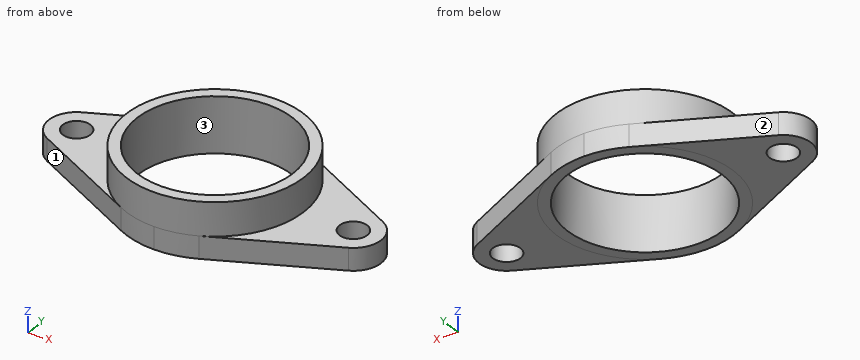
from build123d import *

# Parameters (mm, degrees)
SKETCH_R     = 5
PAD_DEPTH    = 8
SKETCH001_R  = 32
PAD001_DEPTH = 20
SKETCH002_R  = 28
POCKET_DEPTH = 20.0010001


with BuildPart() as part:
    # Sketch → Pad (new body)
    with BuildSketch(Plane.XY):
        with BuildLine():
            Line((-54.4, 8.9799777283), (-14.08, 28.7359287304))
            ThreePointArc((0, 32), (-7.2266963623, 31.1733036377), (-14.08, 28.7359287304))
            Line((0, -32), (0, 32))
            ThreePointArc((-14.08, -28.7359287304), (-7.2266963623, -31.1733036377), (0, -32))
            Line((-54.4, -8.9799777283), (-14.08, -28.7359287304))
            ThreePointArc((-54.4, 8.9799777283), (-60, 0), (-54.4, -8.9799777283))
        make_face()
        with Locations((-50, 0)):
            Circle(SKETCH_R, mode=Mode.SUBTRACT)
    pad = extrude(amount=PAD_DEPTH)

    # Mirrored: Pad across Sketch V_Axis
    add(pad.mirror(Plane(origin=(0, 0, 0), x_dir=(0, 0, 1), z_dir=(1, 0, 0))))

    # Sketch001 → Pad001 (join)
    with BuildSketch(Plane.XY):
        Circle(SKETCH001_R)
    extrude(amount=PAD001_DEPTH)

    # Sketch002 → Pocket (cut, through all)
    with BuildSketch(Plane.XY):
        Circle(SKETCH002_R)
    extrude(amount=POCKET_DEPTH, mode=Mode.SUBTRACT)


solid = part.part
Read the model definition and answer for the solid it produces. Units are mm, in the model's axes. Face numbers are marked on the shaded views. Round coordinates to 2 decimals unless told otherwise and drop trailing zeros. Order: outer loops, then holes, each group sorted by start corner. A loop starts at its lowest first (then second) coordinate and runs counter-clockwise, first axis right, second up. Notation, with made-up numbers: (73.25, 58.25) - (97.25, 58.25) arc R18 cw to (97.25, 75.25) - close; hole circle Ø8 at (-6.5, -27.5). An arc over 180 degrees is marked (long way). Use one line per item in the form item = value. Start each with the question number.
(1) The part is cut by section D-D (y = 12). Give the vertices of the cut face in (x, z).
(2) The part is cut by section A-A (y = 0). Give the vertices of the cut face in (x, z), then the cut area to 3 significant figures.
(3) Flat-ended cylindrical pins translate along their axes: pin 1 Ø11.5 at (x, y) = (-50, 0) entering from -Z; pin 2 Ø10 at (y, z) = (11.5, 10) entering from +X; pin 3 Ø1 at (y, z) = (4, 16) entering from -X; pin 4 Ø23 at (x, y) = (-46, -1.5) entering from +Z. Find the tip coordinate at first contact, or state that the pin passes through.
(4) Find the intervals of material crossed by line 1 along Y through (x, z) = (0, 14); line 2 along Z through (x, y) = (48, 12); line 3 along X through (y, z) = (-8, 12), in increasing order. Write a range as from..to.
(5) The part is cut by section B-B (z = 3.75). Give the vertices of the cut face in (x, y).
(6) The part is cut by section C-C (x = 24). Give the vertices of the cut face in (y, z), then the cut area to 3 significant figures.
(7) Determine the mould class of the marked faces 1, 2 and 3 for opening direction Y: +Y half, -Y half, draft (parallel to the pull), parting line (faces both ways), or undercut.
Checked values:
q1.outline = (-48.24, 0) - (-25.3, 0) - (-25.3, 20) - (-29.66, 20) - (-29.66, 8) - (-48.24, 8) - close; (25.3, 0) - (48.24, 0) - (48.24, 8) - (29.66, 8) - (29.66, 20) - (25.3, 20) - close
q2.outline = (-60, 0) - (-55, 0) - (-55, 8) - (-60, 8) - close; (-45, 0) - (-28, 0) - (-28, 20) - (-32, 20) - (-32, 8) - (-45, 8) - close; (28, 0) - (45, 0) - (45, 8) - (32, 8) - (32, 20) - (28, 20) - close; (55, 0) - (60, 0) - (60, 8) - (55, 8) - close
q2.area = 448 mm^2
q3.pin_1 = 0
q3.pin_2 = 57.22
q3.pin_3 = -31.81
q3.pin_4 = 8
q4.line_1 = -32..-28, 28..32
q4.line_2 = 0..8
q4.line_3 = -30.98..-26.83, 26.83..30.98
q5.outline = (-54.4, -8.98) - (-14.08, -28.74) arc R32 ccw to (14.08, -28.74) - (54.4, -8.98) arc R10 ccw to (54.4, 8.98) - (14.08, 28.74) arc R32 ccw to (-14.08, 28.74) - (-54.4, 8.98) arc R10 ccw to start; hole circle Ø10 at (-50, 0); hole circle Ø56 at (0, 0); hole circle Ø10 at (50, 0)
q6.outline = (-23.88, 0) - (-14.42, 0) - (-14.42, 20) - (-21.17, 20) - (-21.17, 8) - (-23.88, 8) - close; (14.42, 0) - (23.88, 0) - (23.88, 8) - (21.17, 8) - (21.17, 20) - (14.42, 20) - close
q6.area = 313 mm^2
q7.face_1 = -Y half
q7.face_2 = +Y half
q7.face_3 = undercut
